Could you check a few things on this drawing? It's one solid part, dimensions in mm from its lowest x, y, z. A direction names the side the tool comes from. Give positions to 0.01 mm unless a question says otherwise; leave off trailing zeros. Order: outer loops, then holes, each group sorted by start corner. A loop starts at its lowest first (then second) coordinate and runs counter-clockwise, first axis right, second up. Notation, with made-up numbers: (88.5, 32.25) -> (114.5, 32.25) arc R32 ccw to (114.5, 65.25) -> close; hole circle Ø9 at (23.5, 39.5). An arc over 180 degrees is marked (long way). Write each question's results on one line, items separated by ' | '. Start each with the question number.
Q1. Imagine slicing it at C-C, the plane y = 21.5. Please give me the cut outline in (x, z), then the cut area to 3 significant figures.
Q2. For the marked faces 1, 2, 3, 4 and 5, which set-ups out of +Z, -Z, +X, -X, +Y, -Y let a thin tool reach every point of the face, with its end or its side?
Q3. I need wall thicknesses on line 1 along Z through (x, y) = (84, 20); line 2 along X through (y, z) = (61, 103); line 3 along Y through (x, z) = (70, 55). Which ranges of each line are inside material? Lowest first, please. Write a range as [from, to].
Q4. Imagine slicing it at D-D, the plane x = 64.5. Please give me the cut outline in (y, z).
Q5. I'm going to push flat-ended pins straight in: pin 1 (4 mm diameter, centred on x = 78, y = 52.5, fed in from +Z); pin 2 (5 mm diameter, centred on x = 100, y = 40, fed in from -Z); pin 3 (4 mm diameter, centred on x = 68.5, z = 18, fed in from +Y). Where does each tip first touch, or does it pass through?
Q6. Imagine slicing it at A-A, the plane y = 12.5. Please give me the cut outline in (x, z).
Q7. Imagine slicing it at B-B, the plane x = 98. Please give me the cut outline in (y, z), then the cut area to 3 significant figures.
Q8. Thinking about a two-plate mould opening in Z: for the marked faces 6, 7 and 8, which applies, pulls with the +Z half, pulls with the -Z half, needs draft (parallel to the pull), parting line crosses it, or undercut?
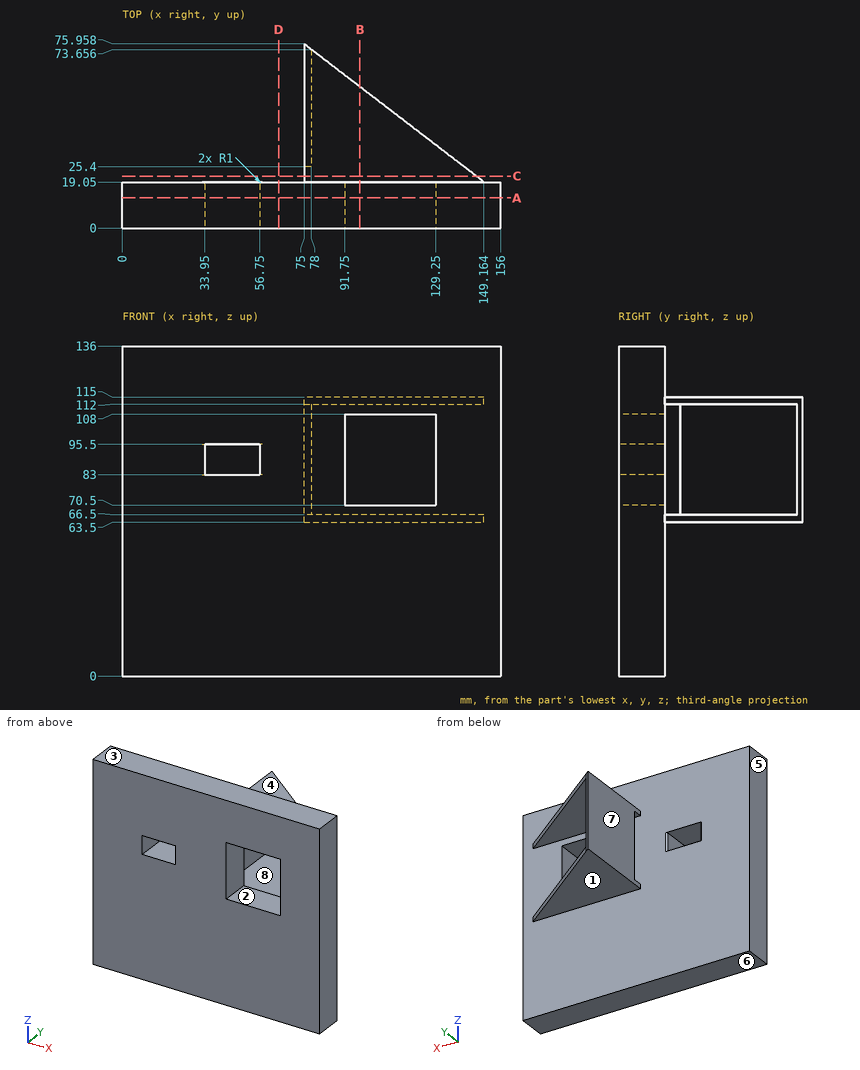
Geometry check:
1) outline: (75, 63.5) -> (145.97, 63.5) -> (145.97, 66.5) -> (75, 66.5) -> close; (75, 112) -> (145.97, 112) -> (145.97, 115) -> (75, 115) -> close | area: 426 mm²
2) face 1: -Z, +X, -X, +Y | face 2: +Y, -Y | face 3: +Z, +X, -X, +Y, -Y | face 4: +Z, +X, -X, +Y | face 5: +Z, -Z, -X, +Y, -Y
3) line 1: [63.5, 66.5], [112, 115] | line 2: [75, 78] | line 3: [0, 19.05]
4) outline: (0, 0) -> (19.05, 0) -> (19.05, 136) -> (0, 136) -> close
5) pin 1: z = 115 | pin 2: z = 63.5 | pin 3: y = 19.05
6) outline: (0, 0) -> (156, 0) -> (156, 136) -> (0, 136) -> close; hole (33.95, 83) -> (56.75, 83) -> (56.75, 95.5) -> (33.95, 95.5) -> close; hole (91.75, 70.5) -> (129.25, 70.5) -> (129.25, 108) -> (91.75, 108) -> close
7) outline: (0, 0) -> (19.05, 0) -> (19.05, 63.5) -> (58.31, 63.5) -> (58.31, 66.5) -> (19.05, 66.5) -> (19.05, 70.5) -> (0, 70.5) -> close; (0, 108) -> (19.05, 108) -> (19.05, 112) -> (58.31, 112) -> (58.31, 115) -> (19.05, 115) -> (19.05, 136) -> (0, 136) -> close | area: 2,110 mm²
8) face 6: pulls with the -Z half | face 7: needs draft | face 8: undercut
